```python
from build123d import *

# Parameters (mm, degrees)
SKETCH1_R                = 32.5
BOSS_EXTRUDE1_DEPTH      = 75
FILLET1_R                = 80
CUT_EXTRUDE3_DEPTH       = 35
FILLET2_R                = 37.5
CUT_EXTRUDE13_DEPTH      = 5
FILLET6_R                = 40
CUT_EXTRUDE14_START      = -27.5
CUT_EXTRUDE14_DEPTH      = 27.5
CUT_EXTRUDE15_START      = -22.5
CUT_EXTRUDE15_DEPTH      = 22.5
SKETCH9_R                = 15
CUT_EXTRUDE16_DEPTH      = 231.204488166
SKETCH10_R               = 20
CUT_EXTRUDE17_DEPTH      = 5
BOSS_EXTRUDE2_DEPTH      = 70
CUT_EXTRUDE20_REACH      = 289.392
CUT_EXTRUDE20_END_RADIUS = 32.5
SKETCH18_W               = 75
SKETCH18_H               = 5


with BuildPart() as part:
    # Sketch1 → Boss-Extrude1 (new body)
    with BuildSketch(Plane.YZ):
        with BuildLine():
            Line((162.308676206, -25), (-102.691323794, -25))
            Line((-102.691323794, -25), (-102.691323794, 25))
            Line((-102.691323794, 25), (62.308676206, 25))
            Line((62.308676206, 25), (62.308676206, 120))
            ThreePointArc((62.308676206, 120), (112.308676206, 170), (162.308676206, 120))
            Line((162.308676206, 120), (162.308676206, -25))
        make_face()
        with Locations(Location((112.308676206, 120, 0), (0, 0, 270))):
            Circle(SKETCH1_R, mode=Mode.SUBTRACT)
    extrude(amount=BOSS_EXTRUDE1_DEPTH)

    # Fillet1
    fillet1_edges = [part.edges().sort_by_distance(p)[0] for p in [
        (37.5, 162.308676206, -25),
    ]]
    fillet(fillet1_edges, radius=FILLET1_R)

    # Sketch3 → Cut-Extrude3 (cut)
    with BuildSketch(Plane.XY.offset(25)):
        with BuildLine():
            Line((75, 62.308676206), (52.5, 62.308676206))
            Line((52.5, 62.308676206), (52.5, -52.14246265))
            ThreePointArc((52.5, -52.14246265), (61.673849507, -62.081213191), (65, -75.191323794))
            ThreePointArc((65, -75.191323794), (56.945436483, -94.636760276), (37.5, -102.691323794))
            Line((37.5, -102.691323794), (75, -102.691323794))
            Line((75, -102.691323794), (75, 62.308676206))
        make_face()
        with BuildLine():
            Line((22.5, -52.14246265), (22.5, 62.308676206))
            Line((22.5, 62.308676206), (0, 62.308676206))
            Line((0, 62.308676206), (0, -102.691323794))
            Line((0, -102.691323794), (37.5, -102.691323794))
            ThreePointArc((37.5, -102.691323794), (11.136258977, -83.014568599), (22.5, -52.14246265))
        make_face()
    extrude(amount=-CUT_EXTRUDE3_DEPTH, mode=Mode.SUBTRACT)

    # Fillet2
    fillet2_edges = [part.edges().sort_by_distance(p)[0] for p in [
        (0, -102.691323794, -17.5),
        (75, -102.691323794, -17.5),
    ]]
    fillet(fillet2_edges, radius=FILLET2_R - 0.0001)  # a hair under: the kernel refuses the full size

    # Sketch7 → Cut-Extrude13 (cut)
    with BuildSketch(Plane.XY.offset(25)):
        with BuildLine():
            Line((52.5, 62.308676206), (22.5, 62.308676206))
            Line((22.5, 62.308676206), (22.5, -52.14246265))
            ThreePointArc((22.5, -52.14246265), (37.5, -47.691323794), (52.5, -52.14246265))
            Line((52.5, -52.14246265), (52.5, 62.308676206))
        make_face()
    extrude(amount=-CUT_EXTRUDE13_DEPTH, mode=Mode.SUBTRACT)

    # Fillet6
    fillet6_edges = [part.edges().sort_by_distance(p)[0] for p in [
        (37.5, 62.308676206, 20),
    ]]
    fillet(fillet6_edges, radius=FILLET6_R)

    # Sketch5 → Cut-Extrude14 (cut)
    with BuildSketch(Plane.YZ.offset(75).offset(CUT_EXTRUDE14_START)):
        with BuildLine():
            ThreePointArc((77.308676206, 60), (72.970807341, 41.454593742), (62.308676206, 25.672700343))
            Line((62.308676206, 25.672700343), (62.308676206, 25))
            Line((62.308676206, 25), (62.308676206, -10))
            Line((62.308676206, -10), (82.308676206, -10))
            ThreePointArc((82.308676206, -10), (128.270616984, 9.038059223), (147.308676206, 55))
            Line((147.308676206, 55), (147.308676206, 84.292857857))
            ThreePointArc((147.308676206, 84.292857857), (112.308676206, 70), (77.308676206, 84.292857857))
            Line((77.308676206, 84.292857857), (77.308676206, 60))
        make_face()
        with BuildLine():
            Line((22.308676206, 10), (-52.14246265, 10))
            Line((-52.14246265, 10), (-52.14246265, -10))
            Line((-52.14246265, -10), (62.308676206, -10))
            Line((62.308676206, -10), (62.308676206, 25))
            Line((62.308676206, 25), (62.308676206, 25.672700343))
            ThreePointArc((62.308676206, 25.672700343), (43.98309625, 13.562881), (22.308676206, 10))
        make_face()
    cut_extrude14 = extrude(amount=CUT_EXTRUDE14_DEPTH, mode=Mode.SUBTRACT)

    # Sketch8 → Cut-Extrude15 (cut)
    with BuildSketch(Plane.YZ.offset(75).offset(CUT_EXTRUDE15_START)):
        with BuildLine():
            ThreePointArc((62.308676206, 120), (66.21095392, 100.635083269), (77.308676206, 84.292857857))
            Line((77.308676206, 84.292857857), (77.308676206, 60))
            ThreePointArc((77.308676206, 60), (72.970807341, 41.454593742), (62.308676206, 25.672700343))
            Line((62.308676206, 25.672700343), (62.308676206, 120))
        make_face()
    cut_extrude15 = extrude(amount=CUT_EXTRUDE15_DEPTH, mode=Mode.SUBTRACT)

    # Mirror2: Cut-Extrude14, Cut-Extrude15 across plane
    add(cut_extrude14.mirror(Plane(origin=(37.5, 0, 0), x_dir=(0, 0, 1), z_dir=(1, 0, 0))), mode=Mode.SUBTRACT)
    add(cut_extrude15.mirror(Plane(origin=(37.5, 0, 0), x_dir=(0, 0, 1), z_dir=(1, 0, 0))), mode=Mode.SUBTRACT)

    # Sketch9 → Cut-Extrude16 (cut, through all)
    with BuildSketch(Plane.XY.offset(25)):
        with Locations((37.5, -75.191323794)):
            Circle(SKETCH9_R)
    cut_extrude16 = extrude(amount=-CUT_EXTRUDE16_DEPTH, mode=Mode.SUBTRACT)

    # Sketch10 → Cut-Extrude17 (cut)
    with BuildSketch(Plane.XY.offset(25)):
        with Locations((37.5, -75.191323794)):
            Circle(SKETCH10_R)
    cut_extrude17 = extrude(amount=-CUT_EXTRUDE17_DEPTH, mode=Mode.SUBTRACT)

    # Mirror3: Cut-Extrude16, Cut-Extrude17 across plane
    add(cut_extrude16.mirror(Plane.XY), mode=Mode.SUBTRACT)
    add(cut_extrude17.mirror(Plane.XY), mode=Mode.SUBTRACT)

    # Sketch13 → Boss-Extrude2 (add)
    with BuildSketch(Plane(origin=(0, 77.30867621, 0), x_dir=(-1, 0, 0), z_dir=(0, 1, 0))):
        with BuildLine():
            Line((-57.423893962, 181.743114855), (-59.932978613, 153.06414606))
            Line((-59.932978613, 153.06414606), (-15.067021387, 153.06414606))
            Line((-15.067021387, 153.06414606), (-17.576106038, 181.743114855))
            ThreePointArc((-17.576106038, 181.743114855), (-37.5, 200), (-57.423893962, 181.743114855))
        make_face()
    extrude(amount=BOSS_EXTRUDE2_DEPTH)

    # Sketch20 → CBORE for M14 Hex Head Cap Screw1 (revolve, cut)
    with BuildSketch(Plane(origin=(37.5, 77.30867621, 181.415910965), x_dir=(0, 0, -1), z_dir=(1, 0, 0))):
        Polygon((0, 0), (0, 84.999999996), (6.75, 84.999999996), (6.75, 6.6), (11, 6.6), (11, 2.223614023), (13.65, 0), align=None)
    revolve(axis=Axis((37.5, 70.95867621, 181.415910965), (0, 1, 0)), mode=Mode.SUBTRACT)

    # Cut-Extrude20: up to this cylinder (the profile starts outside it)
    cut_extrude20_end = Plane(origin=(37.5, 112.308676206, 120), z_dir=(-1, 0, 0)) * Cylinder(CUT_EXTRUDE20_END_RADIUS, 644.784, mode=Mode.PRIVATE)
    # Sketch18 → Cut-Extrude20 (cut, up to the surface)
    with BuildSketch(Plane(origin=(0, 0, 200), x_dir=(-1, 0, 0), z_dir=(0, 0, -1)), mode=Mode.PRIVATE) as cut_extrude20_sk1:
        with Locations((-37.5, 112.308676206)):
            Rectangle(SKETCH18_W, SKETCH18_H)
    cut_extrude20_tool1 = extrude(cut_extrude20_sk1.sketch, amount=CUT_EXTRUDE20_REACH, mode=Mode.PRIVATE) - cut_extrude20_end
    add(cut_extrude20_tool1.solids().sort_by_distance((37.5, 112.308676, 200))[0], mode=Mode.SUBTRACT)


solid = part.part
```
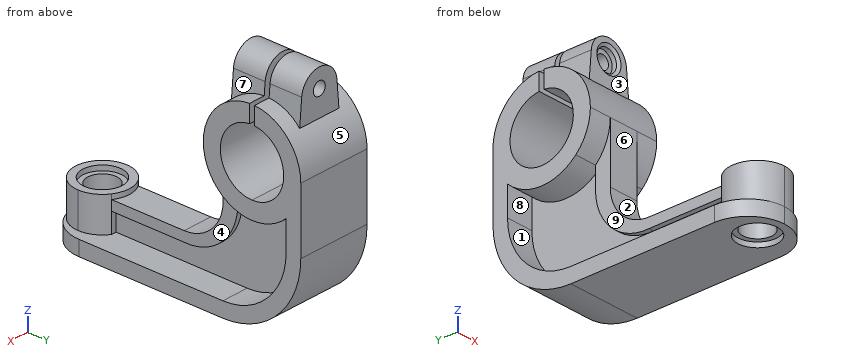
For this review, take the finished solid that the model builds, in its own axes (mm). Face numbers are marked on the shaded views. A direction names the side the tool comes from. Round coordinates to 2 decimals unless told otherwise and drop trailing zeros. Write each loop counter-clockwise with the first axis right and the second up, starting at its lowest first coordinate (ties: lowest second). Pieces come first, ordered by that corner, then holes. Notation, with made-up numbers: (18, 33.25) - (67, 33.25) arc R21 ccw to (67, 61.25) - close; hole circle Ø2 at (63, 63.5). An arc over 180 degrees is marked (long way). Answer as CSV lines item,"result". Start each with the question number.
(1) For line 1 (Y direction, x = 32.5, z = 174); line 2 (Z direction, x = 51, y = 115); line 3 (Z direction, x = 37, y = 135), list the stretches that pass through material, from the lowest coordinate up.
(2) For pin 1 (1 mm diameter, centred on x = 23, z = 112.5, fed in from -Y); pin 2 (4 mm diameter, centred on x = 24, z = 3, fed in from +Y); pin 3 (22 mm diameter, centred on x = 7.5, z = 72.5, fed in from -Y), all flat-tipped, find the tip position at first contact; note any pin that passes through.
(3) Add section B-B, the plane z = 99. State the section outline as (x, y) points, plus the area to 3 significant figures.
(4) Add section D-D, the plane z = 76.5. State the section outline as (x, y) points.
(5) Add section A-A, the plane y = 138. State the section outline as (x, z) points, plus the area to 3 significant figures.
(6) Add section C-C, the plane y = 5. State the section outline as (x, z) points.
(7) Machinability: for the marked faces 1, 2, 3, 4 and 5, which of the approach directions +Z, -Z, +X, -X, +Y, -Y give a long, thin tool a straight path to every point of the face, cutting with its end or side? Answer none if there is none.
(8) Mouldability with a two-part tool opening along Z and no side actions: class the marked faces 6, 7, 8 and 9 as +Z half, -Z half, draft (parallel to the pull), parting line (faces both ways), or undercut.
From the geometry:
1,line 1,"y = 83.91 to 109.81, 114.81 to 147.31"
1,line 2,"z = -18.02 to -1.18, 70.07 to 87.61, 152.39 to 194.76"
1,line 3,"z = -5.2 to 96.73, 143.27 to 174.68, 188.15 to 199.99"
2,pin 1,"stops at y = 62.31"
2,pin 2,"stops at y = 144.76"
2,pin 3,"stops at y = 78.14"
3,outline,"(0, 66.93) - (22.5, 66.93) - (22.5, 62.31) - (52.5, 62.31) - (52.5, 66.93) - (75, 66.93) - (75, 87.5) - (0, 87.5) - close; (0, 137.11) - (75, 137.11) - (75, 162.31) - (0, 162.31) - close"
3,area,"3,570 mm²"
4,outline,"(0, 87.66) - (27.5, 87.66) - (27.5, 77.31) - (22.5, 77.31) - (22.5, 62.31) - (52.5, 62.31) - (52.5, 77.31) - (47.5, 77.31) - (47.5, 87.66) - (75, 87.66) - (75, 136.96) - (47.5, 136.96) - (47.5, 147.31) - (75, 147.31) - (75, 162.31) - (0, 162.31) - (0, 147.31) - (27.5, 147.31) - (27.5, 136.96) - (0, 136.96) - close"
5,outline,"(0, -2.43) - (75, -2.43) - (75, 21.48) - (47.5, 21.48) - (47.5, 77.11) - (75, 77.11) - (75, 100.1) - (0, 100.1) - (0, 77.11) - (27.5, 77.11) - (27.5, 21.48) - (0, 21.48) - close; (0, 139.9) - (75, 139.9) - (75, 162.89) - (59.07, 162.89) - (57.42, 181.74) arc R20 ccw to (17.58, 181.74) - (15.93, 162.89) - (0, 162.89) - close; hole circle Ø13.5 at (37.5, 181.42)"
5,area,"7,550 mm²"
6,outline,"(0, -25) - (75, -25) - (75, -10) - (47.5, -10) - (47.5, 10) - (52.5, 10) - (52.5, 20) - (22.5, 20) - (22.5, 10) - (27.5, 10) - (27.5, -10) - (0, -10) - close"
7,face 1,"-X"
7,face 2,"+Z, +X, -X"
7,face 3,"+Z, +X, -X, -Y"
7,face 4,"+X"
7,face 5,"+Z, +Y"
8,face 6,"draft"
8,face 7,"+Z half"
8,face 8,"undercut"
8,face 9,"undercut"
